from build123d import *

# Parameters (mm, degrees)
SKETCH1_R           = 73.025
SKETCH1_R_2         = 42.926
BOSS_EXTRUDE1_DEPTH = 7.874
SKETCH2_R           = 73.025
SKETCH2_R_2         = 65.151
BOSS_EXTRUDE2_DEPTH = 30.226
BOSS_EXTRUDE3_START = -7.874
SKETCH3_R           = 5.588
BOSS_EXTRUDE3_DEPTH = 7.874
SKETCH4_R           = 5.588
CUT_EXTRUDE1_DEPTH  = 108.605354541


with BuildPart() as part:
    # Sketch1 → Boss-Extrude1 (new body)
    with BuildSketch(Plane(origin=(0, 0, 0), x_dir=(1, 0, 0), z_dir=(0, 1, 0))):
        with Locations(Location((0, 0, 0), (0, 0, 270))):
            Circle(SKETCH1_R)
        with Locations(Location((0, 0, 0), (0, 0, 270))):
            Circle(SKETCH1_R_2, mode=Mode.SUBTRACT)
    extrude(amount=BOSS_EXTRUDE1_DEPTH)

    # Sketch2 → Boss-Extrude2 (add)
    with BuildSketch(Plane(origin=(0, 7.874, 0), x_dir=(1, 0, 0), z_dir=(0, 1, 0))):
        with Locations(Location((0, 0, 0), (0, 0, 270))):
            Circle(SKETCH2_R)
        with Locations(Location((0, 0, 0), (0, 0, 270))):
            Circle(SKETCH2_R_2, mode=Mode.SUBTRACT)
    extrude(amount=BOSS_EXTRUDE2_DEPTH)

    # Sketch3 → Boss-Extrude3 (add)
    # profile 1 of 4: a face of its own
    with BuildSketch(Plane(origin=(0, 38.1, 0), x_dir=(1, 0, 0), z_dir=(0, 1, 0)).offset(BOSS_EXTRUDE3_START)):
        with BuildLine():
            Line((-54.025277323, 11.176), (-64.185277323, 11.176))
            ThreePointArc((-64.185277323, 11.176), (-65.151, 0), (-64.185277323, -11.176))
            Line((-64.185277323, -11.176), (-54.025277323, -11.176))
            ThreePointArc((-54.025277323, -11.176), (-42.849277323, 0), (-54.025277323, 11.176))
        make_face()
        with Locations(Location((-54.025277323, 0, 0), (0, 0, 270))):
            Circle(SKETCH3_R, mode=Mode.SUBTRACT)
    # profile 2 of 4: a face of its own
    with BuildSketch(Plane(origin=(0, 38.1, 0), x_dir=(1, 0, 0), z_dir=(0, 1, 0)).offset(BOSS_EXTRUDE3_START)):
        with BuildLine():
            ThreePointArc((11.176, 64.185277323), (0, 65.151), (-11.176, 64.185277323))
            Line((-11.176, 64.185277323), (-11.176, 54.025277323))
            ThreePointArc((-11.176, 54.025277323), (0, 42.849277323), (11.176, 54.025277323))
            Line((11.176, 54.025277323), (11.176, 64.185277323))
        make_face()
        with Locations(Location((0, 54.025277323, 0), (0, 0, 270))):
            Circle(SKETCH3_R, mode=Mode.SUBTRACT)
    # profile 3 of 4: a face of its own
    with BuildSketch(Plane(origin=(0, 38.1, 0), x_dir=(1, 0, 0), z_dir=(0, 1, 0)).offset(BOSS_EXTRUDE3_START)):
        with BuildLine():
            ThreePointArc((65.151, 0), (64.909120329, 5.608823323), (64.185277323, 11.176))
            Line((64.185277323, 11.176), (54.025277323, 11.176))
            ThreePointArc((54.025277323, 11.176), (42.849277323, 0), (54.025277323, -11.176))
            Line((54.025277323, -11.176), (64.185277323, -11.176))
            ThreePointArc((64.185277323, -11.176), (64.909120329, -5.608823323), (65.151, 0))
        make_face()
        with Locations(Location((54.025277323, 0, 0), (0, 0, 270))):
            Circle(SKETCH3_R, mode=Mode.SUBTRACT)
    # profile 4 of 4: a face of its own
    with BuildSketch(Plane(origin=(0, 38.1, 0), x_dir=(1, 0, 0), z_dir=(0, 1, 0)).offset(BOSS_EXTRUDE3_START)):
        with BuildLine():
            Line((-11.176, -54.025277323), (-11.176, -64.185277323))
            ThreePointArc((-11.176, -64.185277323), (0, -65.151), (11.176, -64.185277323))
            Line((11.176, -64.185277323), (11.176, -54.025277323))
            ThreePointArc((11.176, -54.025277323), (0, -42.849277323), (-11.176, -54.025277323))
        make_face()
        with Locations(Location((0, -54.025277323, 0), (0, 0, 270))):
            Circle(SKETCH3_R, mode=Mode.SUBTRACT)
    extrude(amount=BOSS_EXTRUDE3_DEPTH)

    # Sketch4 → Cut-Extrude1 (cut, through all)
    with BuildSketch(Plane(origin=(0, 7.874, 0), x_dir=(1, 0, 0), z_dir=(0, 1, 0))):
        with Locations(Location((-54.025277323, 0, 0), (0, 0, 270))):
            Circle(SKETCH4_R)
        with Locations(Location((-38.20163995, 38.20163995, 0), (0, 0, 270))):
            Circle(SKETCH4_R)
        with Locations(Location((0, 54.025277323, 0), (0, 0, 270))):
            Circle(SKETCH4_R)
        with Locations(Location((38.20163995, 38.20163995, 0), (0, 0, 270))):
            Circle(SKETCH4_R)
        with Locations(Location((54.025277323, 0, 0), (0, 0, 270))):
            Circle(SKETCH4_R)
        with Locations(Location((38.20163995, -38.20163995, 0), (0, 0, 270))):
            Circle(SKETCH4_R)
        with Locations(Location((0, -54.025277323, 0), (0, 0, 270))):
            Circle(SKETCH4_R)
        with Locations(Location((-38.20163995, -38.20163995, 0), (0, 0, 270))):
            Circle(SKETCH4_R)
    extrude(amount=-CUT_EXTRUDE1_DEPTH, mode=Mode.SUBTRACT)


solid = part.part
Check sheet for the modelled part. Datum: model origin and axes. Units: mm. A direction names the side the tool comes from. Round coordinates to 2 decimals unless told otherwise and drop trailing zeros. Loops run counter-clockwise (first coordinate to the right, second up) from the corner with the lowest first, then second, coordinate; pieces in that order, holes last. Notation, with made-up numbers: (54.25, -10) -> (100.25, -10) arc R16 cw to (100.25, -3) -> close; hole circle Ø7 at (-23.5, 34). An arc over 180 degrees is marked (long way). Put each result on its own line as item: value. Start each with the question number.
1. Section check C-C (y = 33.5). Enter the section's corners in (x, z) (3 decimals), plus the area to 3 significant figures.
2. Scan lines: probe 1 along X at (y, z) = (5.5, 0) (3 decimals); probe 2 along Z at (x, y) = (-4.5, 4.5); probe 3 along X at (y, z) = (3.5, 5). Record each from-to range of solid material in increasing order.
3. Draft check along Z on faces 1 (the face through (-3, 30.226, -59)), 2 (the face through (0, 38.1, 43)), 3 (the face through (21.935, 18.783, 69.653)). Enter one of: +Z half, -Z half, draft (parallel to the pull), parting line (faces both ways), or undercut.
4. Section check A-A (z = 0). Give the number of separate pieces and of enclosed holes in the cut face, plus the area to 3 significant figures.
5. Section check D-D (z = 52). Enter the section's corners in (x, y).
6. Access from +Z, -Z, +X, -X, +Y, -Y to the whole of each face (thin tool, end or side, straight path). Record for faces 4 (the face through (-31, 0, 31)), 5 (the face through (-0.246, 34.108, -42.852)), 6 (the face through (0, 30.226, 61)).
7. Gauge pin test, flat ends, axial feed: pin 1 (13 mm diameter, centred on x = 38.2, z = -38.2, fed in from +Y); pin 2 (6 mm diameter, centred on x = 51.5, y = 26, fed in from +Z); pin 3 (6.5 mm diameter, centred on y = 34.5, z = 61.5, fed in from +X). Record the tip position at first contact, or that the pin passes through.
Findings:
1. outline: circle Ø146.05 at (0, 0); hole (-64.185, -11.176) arc R65.151 ccw to (-11.176, -64.185) -> (-11.176, -54.025) arc R11.176 cw to (11.176, -54.025) -> (11.176, -64.185) arc R65.151 ccw to (64.185, -11.176) -> (54.025, -11.176) arc R11.176 cw to (54.025, 11.176) -> (64.185, 11.176) arc R65.151 ccw to (11.176, 64.185) -> (11.176, 54.025) arc R11.176 cw to (-11.176, 54.025) -> (-11.176, 64.185) arc R65.151 ccw to (-64.185, 11.176) -> (-54.025, 11.176) arc R11.176 cw to (-54.025, -11.176) -> close; hole circle Ø11.176 at (-54.025, 0); hole circle Ø11.176 at (0, -54.025); hole circle Ø11.176 at (0, 54.025); hole circle Ø11.176 at (54.025, 0)
1. area: 4,780 mm^2
2. probe 1: x = -73.025 to -59.613, -48.437 to -42.926, 42.926 to 48.437, 59.613 to 73.025
2. probe 2: z = -72.89 to -57.34, -50.71 to -42.69, 42.69 to 50.71, 57.34 to 72.89
2. probe 3: x = -72.85 to -56.52, -51.53 to -42.63, 42.63 to 51.53, 56.52 to 72.85
3. face 1: undercut
3. face 2: draft
3. face 3: parting line
4. separate pieces: 6
4. enclosed holes: 0
4. area: 949 mm^2
5. outline: (-51.27, 0) -> (-5.21, 0) -> (-5.21, 7.87) -> (-39.25, 7.87) -> (-39.25, 38.1) -> (-51.27, 38.1) -> close; (-10.99, 30.23) -> (-5.21, 30.23) -> (-5.21, 38.1) -> (-10.99, 38.1) -> close; (5.21, 0) -> (51.27, 0) -> (51.27, 38.1) -> (39.25, 38.1) -> (39.25, 7.87) -> (5.21, 7.87) -> close; (5.21, 30.23) -> (10.99, 30.23) -> (10.99, 38.1) -> (5.21, 38.1) -> close
6. face 4: +Z, -Z, +X, -X, -Y
6. face 5: +Y
6. face 6: none
7. pin 1: stops at y = 7.87
7. pin 2: stops at z = 54.59
7. pin 3: stops at x = 44.04
